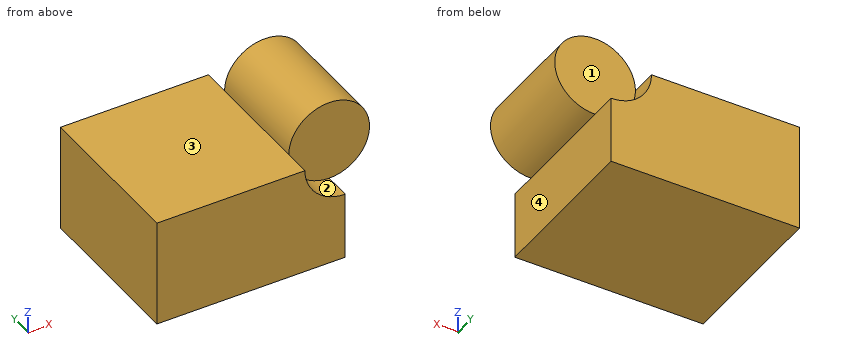
from build123d import *

# Parameters (mm, degrees)
F1_DEPTH = 10
F2_DEPTH = 40


with BuildPart() as f1:
    # F0 (on Front) → F1 (new body, symmetric)
    with BuildSketch(Plane.XZ):
        with BuildLine():
            ThreePointArc((35, 5), (24.3933982822, 9.3933982822), (20, 20))
            Line((20, 20), (-35, 20))
            Line((-35, 20), (-35, -20))
            Line((-35, -20), (35, -20))
            Line((35, -20), (35, 5))
        make_face()
    extrude(amount=F1_DEPTH, both=True)

    # F0 (on Front) + F1_face (on face) → F2 (join)
    with BuildSketch(Plane.XZ):
        with BuildLine():
            Line((35, 5), (35, 20))
            Line((35, 20), (20, 20))
            ThreePointArc((20, 20), (24.3933982822, 9.3933982822), (35, 5))
        make_face()
        with BuildLine():
            Line((20, 20), (35, 20))
            Line((35, 20), (35, 5))
            ThreePointArc((35, 5), (45.6066017178, 9.3933982822), (50, 20))
            ThreePointArc((50, 20), (35, 35), (20, 20))
        make_face()
        with BuildLine():
            ThreePointArc((35, 5), (24.3933982822, 9.3933982822), (20, 20))
            Line((20, 20), (-35, 20))
            Line((-35, 20), (-35, -20))
            Line((-35, -20), (35, -20))
            Line((35, -20), (35, 5))
        make_face()
    with BuildSketch(Plane(origin=(-1.9288829615, -10, -0.9184253163), x_dir=(1, 0, 0), z_dir=(0, -1, 0))):
        with BuildLine():
            ThreePointArc((36.9288829615, 5.9184253163), (26.3222812437, 10.3118235985), (21.9288829615, 20.9184253163))
            Line((21.9288829615, 20.9184253163), (-33.0711170385, 20.9184253163))
            Line((-33.0711170385, 20.9184253163), (-33.0711170385, -19.0815746837))
            Line((-33.0711170385, -19.0815746837), (36.9288829615, -19.0815746837))
            Line((36.9288829615, -19.0815746837), (36.9288829615, 5.9184253163))
        make_face()
    extrude(amount=F2_DEPTH)


solid = f1.part
Check sheet for the modelled part. Datum: model origin and axes. Units: mm. Face numbers are marked on the shaded views. A direction names the side the tool comes from. Round coordinates to 2 decimals unless told otherwise and drop trailing zeros. Loops run counter-clockwise (first coordinate to the right, second up) from the corner with the lowest first, then second, coordinate; pieces in that order, holes last.
1. Sectioned sample at D-D on y = 4.5. Record the boundary of the cut face in (x, z).
2. Scan lines: probe 1 along Z at (x, y) = (-0.5, -5); probe 2 along X at (y, z) = (-33, -7.5); probe 3 along Z at (x, y) = (23, -33.5). Record each from-to range of solid material in increasing order.
3. Gauge pin test, flat ends, axial feed: pin 1 Ø8 at (y, z) = (-21, -7.5) entering from +X; pin 2 Ø9 at (x, z) = (30, 22.5) entering from +Y; pin 3 Ø5 at (x, y) = (-18.5, 3) entering from +Z. Record the tip position at first contact, or that the pin passes through.
4. Sectioned sample at B-B on x = 25.5. Record the boundary of the cut face in (y, z), and give its area (3 significant figures).
5. Set-up check for the marked faces 1, 2, 3 and 4: record each of +Z, -Z, +X, -X, +Y, -Y from which the full face is reachable in a straight line by a thin tool's end or side.
6. Sectioned sample at C-C on z = 14. Record the boundary of the cut face in (x, y), and give its area (3 significant figures).
7. Sectioned sample at A-A on y = -5.5. Record the boundary of the cut face in (x, z).
Recorded:
1. outline: (-35, -20) - (35, -20) - (35, 5) arc R15 cw to (20, 20) - (-35, 20) - close
2. probe 1: z = -20 to 20
2. probe 2: x = -35 to 35
2. probe 3: z = -20 to 29
3. pin 1: stops at x = 35
3. pin 2: stops at y = 0
3. pin 3: stops at z = 20
4. outline: (-50, -20) - (10, -20) - (10, 8.39) - (0, 8.39) - (0, 31.61) - (-40, 31.61) - (-40, 8.39) - (-50, 8.39) - close
4. area: 2,630 mm2
5. face 1: +Z, +X, +Y
5. face 2: +Z, +X, -Y
5. face 3: +Z, -X, +Y, -Y
5. face 4: -Z, +X, +Y, -Y
6. outline: (-35, -50) - (21.25, -50) - (21.25, -40) - (48.75, -40) - (48.75, 0) - (21.25, 0) - (21.25, 10) - (-35, 10) - close
6. area: 4,470 mm2
7. outline: (-35, -20) - (35, -20) - (35, 5) arc R15 ccw (long way) to (20, 20) - (-35, 20) - close
